Here's how the part is built. I have some questions about the finished solid (model axes, mm). Face numbers are marked on the shaded views. A direction names the side the tool comes from. Give positions to 0.01 mm unless a question says otherwise; leave off trailing zeros. Write each loop counter-clockwise with the first axis right and the second up, starting at its lowest first coordinate (ties: lowest second). Pieces come first, ordered by that corner, then holes. Notation, with made-up numbers: (54, 37) - (104, 37) arc R18 ccw to (104, 48) - close; hole circle Ø1 at (-16.75, 68.25). An arc over 180 degrees is marked (long way). One line per item, written item: value. Start each with the question number.
1) Imagine slicing it at B-B on y = 4.5. Write out the boundary of the cut face in (x, z).
2) I'm going to push flat-ended pins straight in: P1, Ø4, axis at y = 5, z = -6, coming from the -X side; P2, Ø15, axis at y = 31.5, z = 2.5, coming from the +X side; P3, Ø4, axis at x = -4.5, y = 10, coming from the +Z side. Where does each tip first touch, or does it pass through?
3) Please list where these lines run through material, in increasing order: L1, parallel to Z at x = 0, y = 8; L2, parallel to Z at x = 9.5, y = 16.5; L3, parallel to X at y = 10.5, z = -2.5. Write a range as [from, to].
4) On a 3-axis mill with a long thin cutter (end or side, diameter ignored), from which of +Z, -Z, +X, -X, +Y, -Y can I reach the whole of each face in a straight line? I mean the marked faces 4, 5 and 6. Say none if no direction works.
5) Imagine slicing it at A-A on x = 0. Write out the boundary of the cut face in (y, z), plus the area to 3 significant figures.
6) We'd pull the mould along Z, two halves only. Please class the marked faces 1, 2 and 3: +Z half, -Z half, draft (parallel to the pull), parting line (faces both ways), or undercut.
Autodesk Inventor part; units mm, degrees
ref_plane "YZ Plane" through (0, 0, 0) normal (1, 0, 0) x (0, 1, 0)
ref_plane "XZ Plane" through (0, 0, 0) normal (0, 1, 0) x (-1, 0, 0)
ref_plane "XY Plane" through (0, 0, 0) normal (0, 0, 1) x (1, 0, 0)
sketch "Boceto1" plane through (0, 0, 0) normal (0, 1, 0) x (-1, 0, 0)
  circle A0 centre (0, 0) radius 16.5
  dimension "d0" = 33
extrude "Extrusión1" add sketch "Boceto1" along normal blind 18
sketch "Boceto3" plane through (0, 0, 0) normal (1, 0, 0) x (0, 1, 0)
  line L0 (18, -16.5) -> (18, 16.5)
  line L1 (18, -12.5) -> (30, -9.7467)
  arc A0 (30, -9.7467) -> (37.7637, 0) centre (27.7637, 0) ccw
  line L2 (18, 0) -> (51.6641, 0)
  line L3 (18, 12.5) -> (30, 9.7467)
  arc A1 (37.7637, 0) -> (30, 9.7467) centre (27.7637, 0) ccw
  line L4 (18, 12.5) -> (18, -12.5)
  point P0 (0, 0)
  dimension "d5" = 10
  dimension "d6" = 4
  dimension "d7" = 12
extrude "Extrusión2" add sketch "Boceto3" along normal mid plane 8
sketch "Boceto4" plane through (4, 0, 0) normal (1, 0, 0) x (0, 0, -1)
  arc A0 (9.7467, 30) -> (-9.7467, 30) centre (0, 27.7637) ccw
  circle A1 centre (0, 27.7637) radius 3
  point P0 (0, 0)
  dimension "d10" = 6
extrude "Extrusión3" cut sketch "Boceto4" against normal through all
sketch "Boceto6" plane through (0, 0, 0) normal (0, -1, 0) x (1, 0, 0)
  circle A0 centre (0, 0) radius 15
  dimension "d14" = 30
extrude "Extrusión4" cut sketch "Boceto6" against normal blind 14
chamfer "Chaflán1" distance 1 angle 45 10 edges at (16.5, 18, 0) (16.5, 0, 0) (-4, 37.7637, 0) (-4, 24, -11.1234) (-4, 24, 11.1234) (4, 37.7637, 0) (4, 24, 11.1234) (4, 24, -11.1234) (0, 18, 12.5) (0, 18, -12.5)
sketch "Boceto7" plane through (0, 0, 0) normal (0, 0, 1) x (1, 0, 0)
  arc A0 (5, 27.7637) -> (-5, 27.7637) centre (0, 27.7637) ccw
  line L0 (4, 36.7637) -> (4, 29.7764)
  line L1 (-4, 29.7764) -> (-4, 36.7637)
  line L2 (-4, 29.7764) -> (-4, 19.9747)
  line L3 (4, 19.9747) -> (4, 29.7764)
  line L4 (4, 30.7637) -> (-4, 30.7637)
  line L5 (4, 24.7637) -> (-4, 24.7637)
  line L6 (8.3579, 27.7637) -> (-7.6994, 27.7637)
  point P0 (0, 0)
  dimension "d20" = 5
revolve "Revolución1" cut sketch "Boceto7" angle 360 about axis through (8.3579, 27.7637, 0) along (-1, 0, 0) contours L6 L3 L0 A0 | L4 A0 | L0 L3 L6 L2 L1 L4 | L1 L2 L6 A0
properties part number "shocks_fixed" material "Goma"
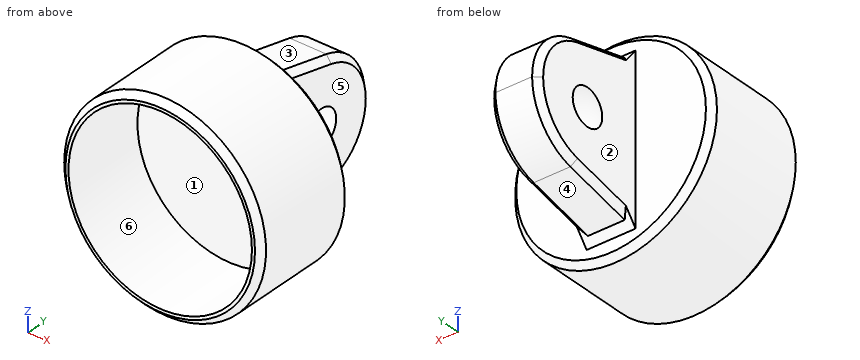
Numbers:
1. outline: circle Ø33 at (0, 0); hole circle Ø30 at (0, 0)
2. P1: x = -16.01
2. P2: x = 4
2. P3: z = 16.31
3. L1: [-16.5, -15], [15, 16.5]
3. L2: [-13.49, 13.49]
3. L3: [-16.31, -14.79], [14.79, 16.31]
4. face 4: -Z, +X, -X, +Y
4. face 5: +Z, -Z, +X, +Y
4. face 6: -Y
5. outline: (0, -15.5) - (1, -16.5) - (17, -16.5) - (18, -15.5) - (18, -13.5) - (18.97, -12.28) - (30, -9.75) arc R10 ccw to (37.76, 0) arc R10 ccw to (30, 9.75) - (18.97, 12.28) - (18, 13.5) - (18, 15.5) - (17, 16.5) - (1, 16.5) - (0, 15.5) - (0, 15) - (14, 15) - (14, -15) - (0, -15) - close; hole circle Ø10 at (27.76, 0)
5. area: 474 mm^2
6. face 1: undercut
6. face 2: draft
6. face 3: +Z half
